Input: part model. Units: mm. Frame: model coordinates. A direction names the side the tool comes from. Give positions to 0.01 mm unless a question says otherwise; leave off trailing zeros. Loops run counter-clockwise (first coordinate to the right, second up) from the corner with the lowest first, then second, coordinate; pieces in that order, holes last. Notation, with made-up numbers: (53.25, 21.25) - (72.25, 21.25) arc R35 ccw to (72.25, 56.25) - close; hole circle Ø8 at (51, 25.25). An arc over 180 degrees is marked (long way). One line per item, written item: value.
from build123d import *

# Parameters (mm, degrees)
RESSALTO_EXTRUS_O1_DEPTH = 5
ESBO_O2_R                = 1.5
ESBO_O2_W                = 20
ESBO_O2_H                = 20
CORTE_EXTRUS_O1_DEPTH    = 29.722813233


with BuildPart() as part:
    # Esboço1 → Ressalto-extrusão1 (new body)
    with BuildSketch(Plane.XY):
        Polygon((20, 0), (20, 20), (-20, 20), (-20, -20), (20, -20), align=None)
    extrude(amount=RESSALTO_EXTRUS_O1_DEPTH)

    # Esboço2 → Corte-extrusão1 (cut, through all)
    with BuildSketch(Plane.XY.offset(5)):
        with Locations((-15, 15)):
            Circle(ESBO_O2_R)
        with Locations((15, 15)):
            Circle(ESBO_O2_R)
        with Locations((-15, -15)):
            Circle(ESBO_O2_R)
        with Locations((15, -15)):
            Circle(ESBO_O2_R)
        Rectangle(ESBO_O2_W, ESBO_O2_H)
    extrude(amount=-CORTE_EXTRUS_O1_DEPTH, mode=Mode.SUBTRACT)


solid = part.part
Item 1: Section D-D, the plane y = -3.5. Output: boundary loops of the cut face in (x, z), and give its area (3 significant figures).
Verdict:
outline: (-20, 0) - (-10, 0) - (-10, 5) - (-20, 5) - close; (10, 0) - (20, 0) - (20, 5) - (10, 5) - close
area: 100 mm^2
Item 2: Material intervals for L1, parallel to Y at x = 15, z = 2.4; L2, parallel to Y at x = -8, z = 0.4, sorted ascending.
Verdict:
L1: y = -20 to -16.5, -13.5 to 13.5, 16.5 to 20
L2: y = -20 to -10, 10 to 20
Item 3: Access query for faces 1 (the face through (0, 10, 3)), 2 (the face through (20, 0, 2)). Directions: +Z, -Z, +X, -X, +Y, -Y. A direction counts if a zero-diameter tool reaches every point of the face in a straight line with its end or side. Return the directions, or none.
Verdict:
face 1: +Z, -Z
face 2: +Z, -Z, +X, +Y, -Y
Item 4: Section A-A, the plane x = 15. Output: boundary loops of the cut face in (y, z).
Verdict:
outline: (-20, 0) - (-16.5, 0) - (-16.5, 5) - (-20, 5) - close; (-13.5, 0) - (13.5, 0) - (13.5, 5) - (-13.5, 5) - close; (16.5, 0) - (20, 0) - (20, 5) - (16.5, 5) - close
Item 5: Pin query (flat end, axial travel): P1, Ø3.5, axis at x = 15, y = 15, coming from the +Z side; P2, Ø2.5, axis at x = -15, y = 15, coming from the -Z side. Return the tip coordinate at first contact, or that it passes through.
Verdict:
P1: stops at z = 5
P2: passes through
Item 6: Draft query along X for faces 3 (the face through (0, 14, 5)), 4 (the face through (-10, 0, 3)), 5 (the face through (-20, 0, 2)). Return one class per face: pulls with the +X half, pulls with the -X half, needs draft (parallel to the pull), parting line crosses it, or undercut.
Verdict:
face 3: needs draft
face 4: undercut
face 5: pulls with the -X half
Item 7: Section C-C, the plane z = 3.4. Output: boundary loops of the cut face in (x, y), and give its area (3 significant figures).
Verdict:
outline: (-20, -20) - (20, -20) - (20, 20) - (-20, 20) - close; hole circle Ø3 at (-15, -15); hole circle Ø3 at (-15, 15); hole (-10, -10) - (10, -10) - (10, 10) - (-10, 10) - close; hole circle Ø3 at (15, -15); hole circle Ø3 at (15, 15)
area: 1,170 mm^2
